The listing builds one solid part. Answer for the finished solid, in the listing's coordinates (mm). Face numbers are marked on the shaded views. A direction names the side the tool comes from. Round coordinates to 2 decimals unless told otherwise and drop trailing zeros. Loops run counter-clockwise (first coordinate to the right, second up) from the corner with the lowest first, then second, coordinate; pieces in that order, holes last. Notation, with made-up numbers: (-31.75, 82) -> (25.25, 82) arc R24 ccw to (25.25, 118) -> close; hole circle Ø6 at (87, -13). An arc over 180 degrees is marked (long way). Write each question's results on one line, items separated by ' | '. Start each with the question number.
(1) The part is cut by section B-B (y = -30.5). Determine the outline of the cut face in (x, z).
(2) Determine the mould class of the marked faces 1, 2 and 3 for opening direction Y: released by +Y, released by -Y, zero draft, split by the parting line, or undercut.
(3) Flat-ended cylindrical pins translate along their axes: pin 1 (5 mm diameter, centred on x = -304, z = -14.5, fed in from -Y); pin 2 (10 mm diameter, centred on x = -277, y = -35.5, fed in from -Z); pin 3 (5.5 mm diameter, centred on x = -302.5, z = -17.5, fed in from -Y). Find the tip coordinate at first contact, or state that the pin passes through.
(4) Straight lines are drawn through the part: probe 1 along Z at (x, y) = (-300.5, -14); probe 2 along Y at (x, z) = (-308, -27); probe 3 along Z at (x, y) = (-290.5, -34.5). For each, find the intervals that lie inside material, in ascending order.
(5) The part is cut by section A-A (z = -7). Determine the outline of the cut face in (x, y).
(6) For the marked faces 4 and 5, determine the directions among +Z, -Z, +X, -X, +Y, -Y from which every point of the face is accessible in a straight line to the end or side of a thin tool.
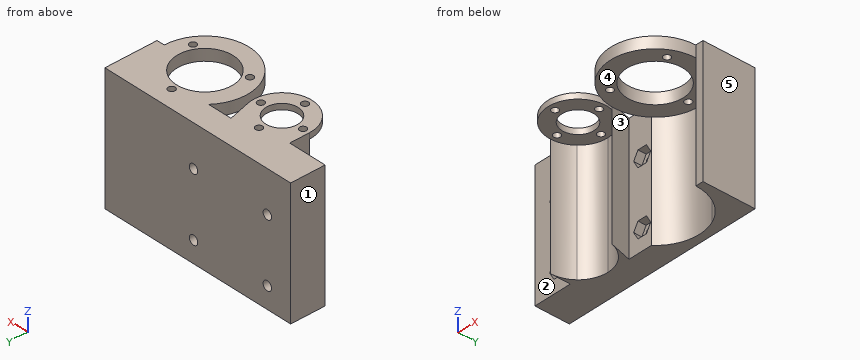
```python
from build123d import *

# Parameters (mm, degrees)
SKETCH1_R           = 1.5
SKETCH1_R_2         = 12.286192875
BOSS_EXTRUDE1_DEPTH = 5
SKETCH1_4_R         = 19.3
SKETCH1_4_R_2       = 1.5
SKETCH1_4_R_3       = 12.286192875
BOSS_EXTRUDE2_DEPTH = 5
SKETCH1_5_R         = 13
SKETCH1_5_R_2       = 1.5
SKETCH1_5_R_3       = 7
BOSS_EXTRUDE3_DEPTH = 2.5
BOSS_EXTRUDE4_DEPTH = 55
SKETCH2_R           = 2
CUT_EXTRUDE1_DEPTH  = 321.699634413
CUT_EXTRUDE2_START  = -7
SKETCH2_3_R         = 2
CUT_EXTRUDE2_DEPTH  = 8


with BuildPart() as part:
    # Sketch1 → Boss-Extrude1 (new body)
    with BuildSketch(Plane.XY):
        with BuildLine():
            Line((-225.050004998, -11.8), (-313.144033158, -11.8))
            Line((-313.144033158, -11.8), (-313.144033158, -26.8))
            Line((-313.144033158, -26.8), (-296.361685959, -26.8))
            Line((-296.361685959, -26.8), (-296.361685959, -35.361873818))
            ThreePointArc((-296.361685959, -35.361873818), (-292.554074115, -26.169485663), (-283.361685959, -22.361873818))
            Line((-283.361685959, -22.361873818), (-262.746762324, -22.361873818))
            ThreePointArc((-262.746762324, -22.361873818), (-254.180514838, -52.695300476), (-228.442241035, -34.500833448))
            Line((-228.442241035, -34.500833448), (-225.050004998, -34.500833448))
            Line((-225.050004998, -34.500833448), (-225.050004998, -11.8))
        make_face()
        with Locations((-234.469948601, -41.489842931)):
            Circle(SKETCH1_R, mode=Mode.SUBTRACT)
        with Locations((-248.325727491, -19.512186292)):
            Circle(SKETCH1_R, mode=Mode.SUBTRACT)
        with Locations((-260.431047012, -42.50047112)):
            Circle(SKETCH1_R, mode=Mode.SUBTRACT)
        with Locations((-247.742241035, -34.500833448)):
            Circle(SKETCH1_R_2, mode=Mode.SUBTRACT)
    extrude(amount=-BOSS_EXTRUDE1_DEPTH)

    # Sketch1<4> → Boss-Extrude2 (add)
    # profile 1 of 3: a face of its own
    with BuildSketch(Plane.XY):
        with Locations((-247.742241035, -34.500833448)):
            Circle(SKETCH1_4_R)
        with Locations((-248.325727491, -19.512186292)):
            Circle(SKETCH1_4_R_2, mode=Mode.SUBTRACT)
        with Locations((-260.431047012, -42.50047112)):
            Circle(SKETCH1_4_R_2, mode=Mode.SUBTRACT)
        with Locations((-234.469948601, -41.489842931)):
            Circle(SKETCH1_4_R_2, mode=Mode.SUBTRACT)
        with Locations((-247.742241035, -34.500833448)):
            Circle(SKETCH1_4_R_3, mode=Mode.SUBTRACT)
    # profile 2 of 3: a face of its own
    with BuildSketch(Plane.XY):
        with BuildLine():
            Line((-225.050004998, -16.8), (-225.050004998, -11.8))
            Line((-225.050004998, -11.8), (-313.144033158, -11.8))
            Line((-313.144033158, -11.8), (-313.144033158, -26.8))
            Line((-313.144033158, -26.8), (-296.361685959, -26.8))
            Line((-296.361685959, -26.8), (-293.144033158, -26.8))
            ThreePointArc((-293.144033158, -26.8), (-288.73270264, -23.523285228), (-283.361685959, -22.361873818))
            Line((-283.361685959, -22.361873818), (-273.361685959, -22.361873818))
            Line((-273.361685959, -22.361873818), (-262.746762324, -22.361873818))
            ThreePointArc((-262.746762324, -22.361873818), (-252.335822317, -15.755460392), (-240.050004998, -16.8))
            Line((-240.050004998, -16.8), (-225.050004998, -16.8))
        make_face()
    # profile 3 of 3: a face of its own
    with BuildSketch(Plane.XY):
        with BuildLine():
            Line((-225.050004998, -34.500833448), (-225.050004998, -16.8))
            Line((-225.050004998, -16.8), (-240.050004998, -16.8))
            ThreePointArc((-240.050004998, -16.8), (-231.603000726, -23.917123217), (-228.442241035, -34.500833448))
            Line((-228.442241035, -34.500833448), (-225.050004998, -34.500833448))
        make_face()
    extrude(amount=-BOSS_EXTRUDE2_DEPTH)

    # Sketch1<5> → Boss-Extrude3 (add)
    with BuildSketch(Plane.XY):
        with Locations((-283.361685959, -35.361873818)):
            Circle(SKETCH1_5_R)
        with Locations((-283.361685959, -25.361873818)):
            Circle(SKETCH1_5_R_2, mode=Mode.SUBTRACT)
        with Locations((-293.361685959, -35.361873818)):
            Circle(SKETCH1_5_R_2, mode=Mode.SUBTRACT)
        with Locations((-283.361685959, -45.361873818)):
            Circle(SKETCH1_5_R_2, mode=Mode.SUBTRACT)
        with Locations((-273.361685959, -35.361873818)):
            Circle(SKETCH1_5_R_2, mode=Mode.SUBTRACT)
        with Locations((-283.361685959, -35.361873818)):
            Circle(SKETCH1_5_R_3, mode=Mode.SUBTRACT)
    extrude(amount=-BOSS_EXTRUDE3_DEPTH)

    # Sketch1<6> → Boss-Extrude4 (add)
    with BuildSketch(Plane.XY):
        with BuildLine():
            Line((-270.796630197, -32.027301328), (-273.361685959, -22.361873818))
            Line((-273.361685959, -22.361873818), (-283.361685959, -22.361873818))
            ThreePointArc((-283.361685959, -22.361873818), (-275.435446068, -25.05776196), (-270.796630197, -32.027301328))
        make_face()
        with BuildLine():
            Line((-225.050004998, -34.500833448), (-225.050004998, -16.8))
            Line((-225.050004998, -16.8), (-240.050004998, -16.8))
            ThreePointArc((-240.050004998, -16.8), (-231.603000726, -23.917123217), (-228.442241035, -34.500833448))
            Line((-228.442241035, -34.500833448), (-225.050004998, -34.500833448))
        make_face()
        with BuildLine():
            Line((-293.144033158, -26.8), (-296.361685959, -26.8))
            Line((-296.361685959, -26.8), (-296.361685959, -35.361873818))
            ThreePointArc((-296.361685959, -35.361873818), (-295.530714548, -30.788609863), (-293.144033158, -26.8))
        make_face()
        with BuildLine():
            Line((-225.050004998, -16.8), (-225.050004998, -11.8))
            Line((-225.050004998, -11.8), (-313.144033158, -11.8))
            Line((-313.144033158, -11.8), (-313.144033158, -26.8))
            Line((-313.144033158, -26.8), (-296.361685959, -26.8))
            Line((-296.361685959, -26.8), (-293.144033158, -26.8))
            ThreePointArc((-293.144033158, -26.8), (-288.73270264, -23.523285228), (-283.361685959, -22.361873818))
            Line((-283.361685959, -22.361873818), (-273.361685959, -22.361873818))
            Line((-273.361685959, -22.361873818), (-262.746762324, -22.361873818))
            ThreePointArc((-262.746762324, -22.361873818), (-252.335822317, -15.755460392), (-240.050004998, -16.8))
            Line((-240.050004998, -16.8), (-225.050004998, -16.8))
        make_face()
    extrude(amount=-BOSS_EXTRUDE4_DEPTH)

    # Sketch2 → Cut-Extrude1 (cut, through all)
    with BuildSketch(Plane(origin=(0, -11.8, 0), x_dir=(1, 0, 0), z_dir=(0, 1, 0))):
        with Locations(Location((-302.09015188, 45.75, 0), (0, 0, 270))):
            Circle(SKETCH2_R)
        with Locations(Location((-302.09015188, 18, 0), (0, 0, 270))):
            Circle(SKETCH2_R)
        with Locations(Location((-267.09015188, 18, 0), (0, 0, 270))):
            Circle(SKETCH2_R)
        with Locations(Location((-267.09015188, 45.75, 0), (0, 0, 270))):
            Circle(SKETCH2_R)
    extrude(amount=-CUT_EXTRUDE1_DEPTH, mode=Mode.SUBTRACT)

    # Sketch2<3> → Cut-Extrude2 (cut)
    # profile 1 of 4: a face of its own
    with BuildSketch(Plane(origin=(0, -11.8, 0), x_dir=(1, 0, 0), z_dir=(0, 1, 0)).offset(CUT_EXTRUDE2_START)):
        Polygon((-300.069425938, 42.25), (-298.048699996, 45.75), (-300.069425938, 49.25), (-304.110877823, 49.25), (-306.131603765, 45.75), (-304.110877823, 42.25), align=None)
        with Locations(Location((-302.09015188, 45.75, 0), (0, 0, 270))):
            Circle(SKETCH2_3_R, mode=Mode.SUBTRACT)
    # profile 2 of 4: a face of its own
    with BuildSketch(Plane(origin=(0, -11.8, 0), x_dir=(1, 0, 0), z_dir=(0, 1, 0)).offset(CUT_EXTRUDE2_START)):
        Polygon((-300.069425938, 14.5), (-298.048699996, 18), (-300.069425938, 21.5), (-304.110877823, 21.5), (-306.131603765, 18), (-304.110877823, 14.5), align=None)
        with Locations(Location((-302.09015188, 18, 0), (0, 0, 270))):
            Circle(SKETCH2_3_R, mode=Mode.SUBTRACT)
    # profile 3 of 4: a face of its own
    with BuildSketch(Plane(origin=(0, -11.8, 0), x_dir=(1, 0, 0), z_dir=(0, 1, 0)).offset(CUT_EXTRUDE2_START)):
        Polygon((-269.110877823, 21.5), (-271.131603765, 18), (-269.110877823, 14.5), (-265.069425938, 14.5), (-263.048699996, 18), (-265.069425938, 21.5), align=None)
        with Locations(Location((-267.09015188, 18, 0), (0, 0, 270))):
            Circle(SKETCH2_3_R, mode=Mode.SUBTRACT)
    # profile 4 of 4: a face of its own
    with BuildSketch(Plane(origin=(0, -11.8, 0), x_dir=(1, 0, 0), z_dir=(0, 1, 0)).offset(CUT_EXTRUDE2_START)):
        Polygon((-269.110877823, 42.25), (-265.069425938, 42.25), (-263.048699996, 45.75), (-265.069425938, 49.25), (-269.110877823, 49.25), (-271.131603765, 45.75), align=None)
        with Locations(Location((-267.09015188, 45.75, 0), (0, 0, 270))):
            Circle(SKETCH2_3_R, mode=Mode.SUBTRACT)
    extrude(amount=-CUT_EXTRUDE2_DEPTH, mode=Mode.SUBTRACT)


solid = part.part
```
Checked values:
1) outline: (-296.36, -55) -> (-295.42, -55) -> (-295.42, -2.5) -> (-288.4, -2.5) -> (-288.4, 0) -> (-296.36, 0) -> close; (-278.33, -2.5) -> (-271.31, -2.5) -> (-271.31, -55) -> (-271.2, -55) -> (-271.2, 0) -> (-278.33, 0) -> close; (-266.62, -5) -> (-259.36, -5) -> (-259.36, 0) -> (-266.62, 0) -> close; (-236.13, -5) -> (-228.86, -5) -> (-228.86, -55) -> (-225.05, -55) -> (-225.05, 0) -> (-236.13, 0) -> close
2) face 1: zero draft | face 2: released by -Y | face 3: undercut
3) pin 1: stops at y = -26.8 | pin 2: stops at z = -2.5 | pin 3: stops at y = -18.8
4) probe 1: z = -55 to -46.96, -44.54 to -19.21, -16.79 to 0 | probe 2: y = -26.8 to -11.8 | probe 3: z = -2.5 to 0
5) outline: (-313.14, -26.8) -> (-296.36, -26.8) -> (-296.36, -35.36) arc R13 cw to (-270.8, -32.03) -> (-273.36, -22.36) -> (-262.75, -22.36) arc R19.3 cw to (-228.44, -34.5) -> (-225.05, -34.5) -> (-225.05, -11.8) -> (-313.14, -11.8) -> close
6) face 4: -Z, -Y | face 5: +Z, -Z, +X, +Y, -Y
